Model file for the job. Use its own axes, mm. A direction names the side the tool comes from. Give positions to 0.01 mm unless a question says otherwise; leave off trailing zeros. Loops run counter-clockwise (first coordinate to the right, second up) from the corner with the lowest first, then second, coordinate; pieces in that order, holes last. Notation, with made-up numbers: (-27, -38) - (21, -38) arc R20 cw to (21, 0) - close; hole circle Ø6 at (38, 33.25). An arc over 180 degrees is marked (long way). Use a Markdown table: item, result.
from build123d import *

# Parameters (mm, degrees)
CUT_EXTRUDE1_START = -0.7874
CUT_EXTRUDE1_DEPTH = 14.3002
CIRPATTERN1_COUNT  = 16
SKETCH4_R          = 3.175
CUT_EXTRUDE2_DEPTH = 43.478219515
CUT_EXTRUDE3_DEPTH = 2.38125


with BuildPart() as part:
    # Sketch2 → Revolve1 (revolve)
    with BuildSketch(Plane(origin=(0, 0, 0), x_dir=(0, 0, -1), z_dir=(1, 0, 0)), mode=Mode.PRIVATE) as revolve1_sk:
        with BuildLine():
            Line((-17.4625, 6.35), (17.4625, 6.35))
            Line((17.4625, 6.35), (17.4625, 27.3812))
            Line((17.4625, 27.3812), (16.27505, 27.3812))
            ThreePointArc((16.27505, 27.3812), (15.408504076, 26.591481572), (15.0876, 25.463839073))
            Line((15.0876, 25.463839073), (15.0876, 23.546478146))
            Line((15.0876, 23.546478146), (0.7874, 23.546478146))
            Line((0.7874, 23.546478146), (0.7874, 25.463839073))
            ThreePointArc((0.7874, 25.463839073), (0.466495924, 26.591481572), (-0.40005, 27.3812))
            Line((-0.40005, 27.3812), (-1.5875, 27.3812))
            Line((-1.5875, 27.3812), (-1.5875, 18.2626))
            Line((-1.5875, 18.2626), (-17.4625, 18.2626))
            Line((-17.4625, 18.2626), (-17.4625, 6.35))
        make_face()
    revolve(revolve1_sk.sketch.rotate(Axis((0, 0, 17.4625), (0, 0, -1)), 90), axis=Axis((0, 0, 17.4625), (0, 0, -1)))

    # Sketch3 → Cut-Extrude1 (cut)
    with BuildSketch(Plane.XY.offset(CUT_EXTRUDE1_START)):
        with BuildLine():
            Line((-1.630736704, 21.5265), (1.630736704, 21.5265))
            Line((1.630736704, 21.5265), (2.3241, 23.4315))
            ThreePointArc((2.3241, 23.4315), (0, 23.546478146), (-2.3241, 23.4315))
            Line((-2.3241, 23.4315), (-1.630736704, 21.5265))
        make_face()
    cut_extrude1 = extrude(amount=-CUT_EXTRUDE1_DEPTH, mode=Mode.SUBTRACT)

    # CirPattern1: Cut-Extrude1 ×16 about axis
    cirpattern1_axis = Axis((0, 0, 0), (0, 0, 1))
    for i in range(1, CIRPATTERN1_COUNT):
        add(cut_extrude1.rotate(cirpattern1_axis, i * 360 / CIRPATTERN1_COUNT), mode=Mode.SUBTRACT)

    # Sketch4 → Cut-Extrude2 (cut, through all)
    with BuildSketch(Plane(origin=(0, 0, 0), x_dir=(0, -1, 0), z_dir=(1, 0, 0))):
        with Locations(Location((0, -9.525, 0), (0, 0, 270))):
            Circle(SKETCH4_R)
    extrude(amount=CUT_EXTRUDE2_DEPTH, mode=Mode.SUBTRACT)

    # Sketch5 → Revolve2 (revolve)
    with BuildSketch(Plane.XY.offset(9.525)):
        Polygon((6.35, -2.794), (6.35, 0), (17.984491479, 0), (17.984491479, -2.794), (17.603491479, -3.175), (6.731, -3.175), align=None)
    revolve(axis=Axis((6.35, 0, 9.525), (1, 0, 0)))

    # Sketch6 → Cut-Extrude3 (cut)
    with BuildSketch(Plane(origin=(17.984491479, 5.384140679, 0), x_dir=(0, -1, 0), z_dir=(-1, 0, 0))):
        Polygon((5.384140679, 11.358087105), (3.796640679, 10.441543552), (3.796640679, 8.608456448), (5.384140679, 7.691912895), (6.971640679, 8.608456448), (6.971640679, 10.441543552), align=None)
    extrude(amount=CUT_EXTRUDE3_DEPTH, mode=Mode.SUBTRACT)


solid = part.part
(1) Mould opens along Y. For faces 4 (the flat face through (-10.44, 20.02, -7.84)), 5 (the flat face through (6.775, -21.51, -7.837)), 6 (the cylindrical face through (19.6, -13.05, -7.84)), 7 (the flat face through (14.5, 17.3, -7.8)) say: pulls with the +Y half, pulls with the -Y half, needs draft (parallel to the pull), parting line crosses it, or undercut.
Computed:
| item | result |
|---|---|
| face 4 | pulls with the +Y half |
| face 5 | undercut |
| face 6 | pulls with the -Y half |
| face 7 | undercut |
(2) 3-axis set-ups, long thin cutter, end or side, ignore diameter. For faces 1 (the flat face through (-1.98, 22.49, -7.84)), 2 (the flat face through (-22.49, -1.98, -7.84)), 3 (the cylindrical face through (6.243, 2.817, 10.99)): which of +Z, -Z, +X, -X, +Y, -Y reach the whole face in a straight line?
Computed:
| item | result |
|---|---|
| face 1 | +Y |
| face 2 | -X |
| face 3 | none |
(3) Drill centre lines: probe 1 along Z at (x, y) = (-5.5, 23.5); probe 2 along Y at (x, z) = (0, 5); probe 3 along X at (y, z) = (0, 10). Where is each one in solid material? Low to high. Write a range as [from, to].
Computed:
| item | result |
|---|---|
| probe 1 | [-17.46, -15.09], [-0.79, 1.59] |
| probe 2 | [-18.26, -6.35], [6.35, 18.26] |
| probe 3 | [-18.26, -6.35], [6.35, 15.6] |
(4) Slice it at A-A, the plane x = 0. Write the cut outline in (y, z), plus the area to 3 significant figures.
Computed:
| item | result |
|---|---|
| outline | (-27.38, -17.46) - (-6.35, -17.46) - (-6.35, 17.46) - (-18.26, 17.46) - (-18.26, 1.59) - (-27.38, 1.59) - (-27.38, 0.4) arc R2.14 ccw to (-25.46, -0.79) - (-21.53, -0.79) - (-21.53, -15.09) - (-25.46, -15.09) arc R2.14 ccw to (-27.38, -16.28) - close; (6.35, -17.46) - (27.38, -17.46) - (27.38, -16.28) arc R2.14 ccw to (25.46, -15.09) - (21.53, -15.09) - (21.53, -0.79) - (25.46, -0.79) arc R2.14 ccw to (27.38, 0.4) - (27.38, 1.59) - (18.26, 1.59) - (18.26, 17.46) - (6.35, 17.46) - close |
| area | 1,010 mm² |
(5) Pin check, flat tips, straight feed: P1, Ø1.6, axis at y = -0.5, z = -8, coming from the -X side; P2, Ø11.5, axis at x = 0, y = 0, coming from the -Z side; P3, Ø0.5, axis at x = 17, z = 9, coming from the -Y side; P4, Ø1.5, axis at x = 3.5, z = -3.5, coming from the +Y side. Stop position of each tip, or through.
Computed:
| item | result |
|---|---|
| P1 | x = -21.53 |
| P2 | through |
| P3 | y = -7.28 |
| P4 | y = 23.39 |
